Design review of the part built by this model. Coordinates are the model's own, in mm. Coordinates: 2 decimals unless noted, no trailing zeros. Loops run counter-clockwise (first coordinate to the right, second up) from the corner with the lowest first, then second, coordinate; pieces in that order, holes last. Notation, with made-up numbers: M 36,-35 L 77,-35 A22 cw 77,-17 Z; hole C 53.5,-8 d5. An arc over 180 degrees is marked long. Put each result on its own line as item: value. Start each with the question number.
(1) Take a section at A-A, the plane y = 0. Give the boundary of the cut face in (x, z).
(2) Clearance check with a flat-ended pin moving along its axis: pin 1 (1 mm diameter, centred on y = -31.5, z = 22.5, fed in from +X). State where the tip first meets the part, or that it passes through.
(3) Take a section at C-C, the plane x = 18. Give the boundary of the cut face in (y, z).
(4) Take a section at D-D, the plane y = -18. Give the boundary of the cut face in (x, z), then the cut area to 3 significant figures.
(5) Take a section at B-B, the plane x = 0. Give the boundary of the cut face in (y, z), then the cut area to 3 significant figures.
(6) For probe 1 along Y at (x, z) = (0, 23); probe 2 along X at (y, z) = (-19, 23.8); probe 3 along Y at (x, z) = (-28, 23.55), list the stretches that pass through material, from the lowest coordinate up. Write a range as [from, to].
```python
from build123d import *

# Parameters (mm, degrees)
SKETCH006_R   = 43
SKETCH006_R_2 = 1.6
SKETCH006_R_3 = 30.5
PAD_DEPTH     = 2


with BuildPart() as part:
    # Sketch006 → Pad (new body)
    with BuildSketch(Plane.XY.offset(22)):
        Circle(SKETCH006_R)
        with Locations((0, 36)):
            Circle(SKETCH006_R_2, mode=Mode.SUBTRACT)
        with Locations((31.176915, -18)):
            Circle(SKETCH006_R_2, mode=Mode.SUBTRACT)
        with Locations((-31.176915, -18)):
            Circle(SKETCH006_R_2, mode=Mode.SUBTRACT)
        Circle(SKETCH006_R_3, mode=Mode.SUBTRACT)
    extrude(amount=PAD_DEPTH)


solid = part.part
```
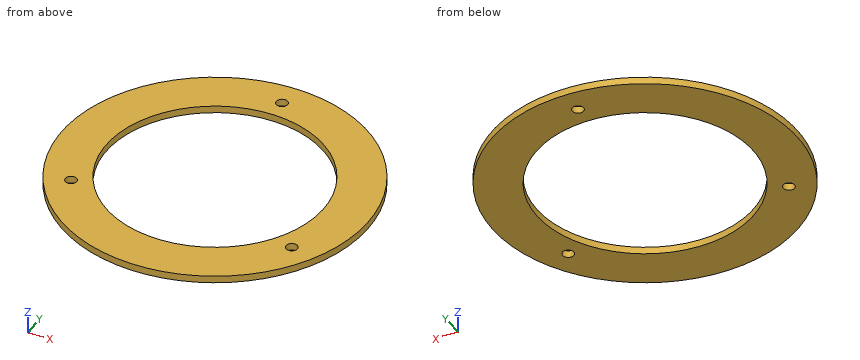
Computed values:
1. outline: M -43,22 L -30.5,22 L -30.5,24 L -43,24 Z; M 30.5,22 L 43,22 L 43,24 L 30.5,24 Z
2. pin 1: stops at x = 29.8
3. outline: M -39.05,22 L -24.62,22 L -24.62,24 L -39.05,24 Z; M 24.62,22 L 39.05,22 L 39.05,24 L 24.62,24 Z
4. outline: M -39.05,22 L -32.78,22 L -32.78,24 L -39.05,24 Z; M -29.58,22 L -24.62,22 L -24.62,24 L -29.58,24 Z; M 24.62,22 L 29.58,22 L 29.58,24 L 24.62,24 Z; M 32.78,22 L 39.05,22 L 39.05,24 L 32.78,24 Z
4. area: 44.9 mm^2
5. outline: M -43,22 L -30.5,22 L -30.5,24 L -43,24 Z; M 30.5,22 L 34.4,22 L 34.4,24 L 30.5,24 Z; M 37.6,22 L 43,22 L 43,24 L 37.6,24 Z
5. area: 43.6 mm^2
6. probe 1: y = [-43, -30.5], [30.5, 34.4], [37.6, 43]
6. probe 2: x = [-38.57, -32.43], [-29.93, -23.86], [23.86, 29.93], [32.43, 38.57]
6. probe 3: y = [-32.63, -12.09], [12.09, 32.63]
